The listing builds one solid part. Answer for the finished solid, in the listing's coordinates (mm). Face numbers are marked on the shaded views. A direction names the side the tool comes from. Give positions to 0.01 mm unless a question says otherwise; leave off trailing zeros. Order: outer loops, then holes, each group sorted by start corner. A loop starts at its lowest first (then second) coordinate and runs counter-clockwise, first axis right, second up. Notation, with made-up numbers: (61.5, -33) - (107.5, -33) arc R20 cw to (107.5, -24) - close; hole circle Ø8 at (36.25, -36). An arc over 180 degrees is marked (long way). Answer in a Markdown table with one row per item.
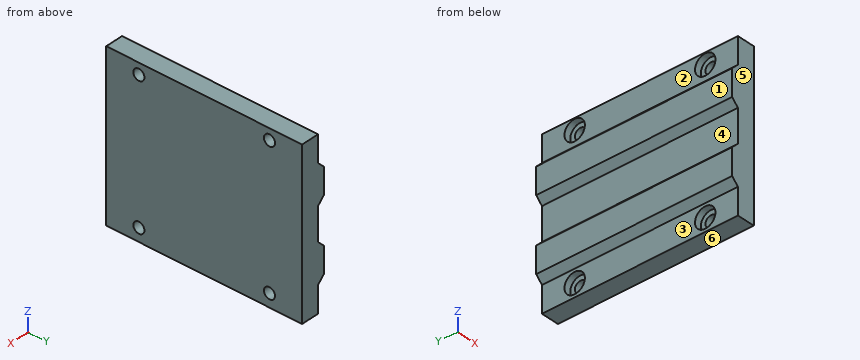
from build123d import *

# Parameters (mm, degrees)
F1_DEPTH = 76.2
F3_D     = 4.318
F3_DEPTH = 12.7
F3_TIP   = 1.2972580765
F4_D     = 4.318
F4_DEPTH = 12.7
F4_TIP   = 1.2972580765
F5_R     = 3.96875
F5_R_2   = 2.159
F6_DEPTH = 2.54
F7_DEPTH = 2.54


with BuildPart() as f1:
    # F0 (on Front) → F1 (new body)
    with BuildSketch(Plane.XZ):
        Polygon((6.985, 50.8), (6.985, 40.64), (9.525, 38.1), (9.525, 25.4), (6.985, 22.86), (6.985, 12.7), (9.525, 10.16), (9.525, 0), (16.51, 0), (16.51, 63.5), (9.525, 63.5), (9.525, 53.34), align=None)
    extrude(amount=F1_DEPTH)

    # F3
    with Locations(Plane(origin=(9.525, 0, 0), x_dir=(0, -1, 0), z_dir=(-1, 0, 0))):
        with Locations((12.7, 5.08), (63.5, 5.08)):
            Hole(F3_D / 2, depth=F3_DEPTH)
            with Locations((0, 0, -(F3_DEPTH + F3_TIP / 2))):  # 118° drill point
                Cone(0, F3_D / 2, F3_TIP, mode=Mode.SUBTRACT)

    # F4
    with Locations(Plane(origin=(9.525, 0, 0), x_dir=(0, -1, 0), z_dir=(-1, 0, 0))):
        with Locations((12.7, 59.182), (63.5, 59.182)):
            Hole(F4_D / 2, depth=F4_DEPTH)
            with Locations((0, 0, -(F4_DEPTH + F4_TIP / 2))):  # 118° drill point
                Cone(0, F4_D / 2, F4_TIP, mode=Mode.SUBTRACT)

    # F5 (on face) → F6 (cut)
    with BuildSketch(Plane(origin=(9.525, 0, 0), x_dir=(0, -1, 0), z_dir=(-1, 0, 0))):
        with Locations((12.7, 5.08)):
            Circle(F5_R)
        with Locations((12.7, 5.08)):
            Circle(F5_R_2, mode=Mode.SUBTRACT)
        with Locations((63.5, 5.08)):
            Circle(F5_R)
        with Locations((63.5, 5.08)):
            Circle(F5_R_2, mode=Mode.SUBTRACT)
    extrude(amount=-F6_DEPTH, mode=Mode.SUBTRACT)

    # F5 (on face) → F7 (cut)
    with BuildSketch(Plane(origin=(9.525, 0, 0), x_dir=(0, -1, 0), z_dir=(-1, 0, 0))):
        with Locations((12.7, 59.182)):
            Circle(F5_R)
        with Locations((12.7, 59.182)):
            Circle(F5_R_2, mode=Mode.SUBTRACT)
        with Locations((63.5, 59.182)):
            Circle(F5_R)
        with Locations((63.5, 59.182)):
            Circle(F5_R_2, mode=Mode.SUBTRACT)
    extrude(amount=-F7_DEPTH, mode=Mode.SUBTRACT)


solid = f1.part
Item 1: Find section B-B on y = -48. Write down the section's boundary in (x, z) (3 decimals), then the cut area to 3 significant figures.
Answer block:
| item | result |
|---|---|
| outline | (6.985, 12.7) - (9.525, 10.16) - (9.525, 0) - (16.51, 0) - (16.51, 63.5) - (9.525, 63.5) - (9.525, 53.34) - (6.985, 50.8) - (6.985, 40.64) - (9.525, 38.1) - (9.525, 25.4) - (6.985, 22.86) - close |
| area | 508 mm² |
Item 2: Which of the six approach directions +Z, -Z, +X, -X, +Y, -Y give full straight-line access (tool end or side, diameter ignored) to the marked faces 1, 2 and 3?
Answer block:
| item | result |
|---|---|
| face 1 | +Z, -Z, -X, +Y, -Y |
| face 2 | +Z, -X, +Y, -Y |
| face 3 | -Z, -X, +Y, -Y |
Item 3: Find section A-A on y = -63.5. Write down the section's boundary in (x, z) (3 decimals).
Answer block:
| item | result |
|---|---|
| outline | (6.985, 12.7) - (9.525, 10.16) - (9.525, 9.049) - (12.065, 9.049) - (12.065, 7.239) - (16.51, 7.239) - (16.51, 57.023) - (12.065, 57.023) - (12.065, 55.213) - (9.525, 55.213) - (9.525, 53.34) - (6.985, 50.8) - (6.985, 40.64) - (9.525, 38.1) - (9.525, 25.4) - (6.985, 22.86) - close; (9.525, 0) - (16.51, 0) - (16.51, 2.921) - (12.065, 2.921) - (12.065, 1.111) - (9.525, 1.111) - close; (9.525, 63.151) - (12.065, 63.151) - (12.065, 61.341) - (16.51, 61.341) - (16.51, 63.5) - (9.525, 63.5) - close |
Item 4: Find section C-C on z = 34.5. Write down the section's boundary in (x, y) (3 decimals), then the cut area to 3 significant figures.
Answer block:
| item | result |
|---|---|
| outline | (9.525, -76.2) - (16.51, -76.2) - (16.51, 0) - (9.525, 0) - close |
| area | 532 mm² |
Item 5: Determine the mould class of the marked faces 4, 5 and 6 for opening direction Z: pulls with the +Z half, pulls with the -Z half, needs draft (parallel to the pull), parting line crosses it, or undercut.
Answer block:
| item | result |
|---|---|
| face 4 | undercut |
| face 5 | needs draft |
| face 6 | pulls with the -Z half |
Item 6: Consider line 1 (Z direction, x = 11.45, y = -12.7); line 2 (Z direction, x = 13.55, y = -63.5); line 3 (Y direction, x = 14.4, z = 5.08). Determine where each line is inside the solid, lowest interval first.
Answer block:
| item | result |
|---|---|
| line 1 | 0 to 1.11, 9.05 to 55.21, 63.15 to 63.5 |
| line 2 | 0 to 2.92, 7.24 to 57.02, 61.34 to 63.5 |
| line 3 | -76.2 to -65.66, -61.34 to -14.86, -10.54 to 0 |
Item 7: Find section D-D on y = -12. Write down the section's boundary in (x, z) (3 decimals), then the cut area to 3 significant figures.
Answer block:
| item | result |
|---|---|
| outline | (6.985, 12.7) - (9.525, 10.16) - (9.525, 8.987) - (12.065, 8.987) - (12.065, 7.122) - (16.51, 7.122) - (16.51, 57.14) - (12.065, 57.14) - (12.065, 55.275) - (9.525, 55.275) - (9.525, 53.34) - (6.985, 50.8) - (6.985, 40.64) - (9.525, 38.1) - (9.525, 25.4) - (6.985, 22.86) - close; (9.525, 0) - (16.51, 0) - (16.51, 3.038) - (12.065, 3.038) - (12.065, 1.173) - (9.525, 1.173) - close; (9.525, 63.089) - (12.065, 63.089) - (12.065, 61.224) - (16.51, 61.224) - (16.51, 63.5) - (9.525, 63.5) - close |
| area | 432 mm² |
Item 8: Each of these flat-tipped pins is pushed along its axis until it touches: P1, Ø11, axis at y = -34.5, z = 56.5, coming from the -X side (3 decimals); P2, Ø12.5, axis at y = -63.5, z = 59.182, coming from the +X side; P3, Ø6.5, axis at y = -19, z = 34.5, coming from the -X side (3 decimals); P4, Ø8.5, axis at y = -65, z = 57.5, coming from the -X side (3 decimals). Where does it stop, or does it pass through?
Answer block:
| item | result |
|---|---|
| P1 | x = 7.185 |
| P2 | x = 16.51 |
| P3 | x = 9.525 |
| P4 | x = 9.435 |
